Geometry: final body of the model. Coordinates: model frame, mm. Face numbers are marked on the shaded views. A direction names the side the tool comes from. Round coordinates to 2 decimals unless told otherwise and drop trailing zeros. Write each loop counter-clockwise with the first axis right and the second up, starting at its lowest first coordinate (ties: lowest second). Pieces come first, ordered by that corner, then holes.
from build123d import *

# Parameters (mm, degrees)
BOSS_EXTRUDE1_DEPTH = 25.5
CUT_EXTRUDE1_DEPTH  = 12.5
CUT_EXTRUDE2_DEPTH  = 15.75
BOSS_EXTRUDE2_REACH = 27.5
SKETCH2_W           = 6.25
SKETCH2_H           = 14
CUT_EXTRUDE3_DEPTH  = 9.5
FILLET1_R           = 8


with BuildPart() as part:
    # Sketch1 → Boss-Extrude1 (new body)
    with BuildSketch(Plane(origin=(0, 0, 0), x_dir=(1, 0, 0), z_dir=(0, 1, 0))):
        Polygon((0, 0), (44, 0), (44, -26), (34.5, -26), (34.5, -32), (0, -32), align=None)
    extrude(amount=BOSS_EXTRUDE1_DEPTH)

    # Sketch3 → Cut-Extrude1 (cut)
    with BuildSketch(Plane.ZY):
        Polygon((32, 25.5), (3.5, 25.5), (32, 9.5), align=None)
    extrude(amount=-CUT_EXTRUDE1_DEPTH, mode=Mode.SUBTRACT)

    # Sketch4 → Cut-Extrude2 (cut)
    with BuildSketch(Plane.ZY.offset(-12.5)):
        Polygon((32, 25.5), (3.5, 25.5), (32, 16), align=None)
    extrude(amount=-CUT_EXTRUDE2_DEPTH, mode=Mode.SUBTRACT)

    # Boss-Extrude2: up to this face of the body (flat: up to its plane)
    boss_extrude2_end = Plane(part.part.faces().sort_by_distance((20.375, 20.75, 17.75))[0])
    # Sketch2 → Boss-Extrude2 (add, up to the picked face)
    with BuildSketch(Plane(origin=(0, 25.5, 0), x_dir=(1, 0, 0), z_dir=(0, 1, 0)), mode=Mode.PRIVATE) as boss_extrude2_sk1:
        with Locations((15.625, -10.5)):
            Rectangle(SKETCH2_W, SKETCH2_H)
    boss_extrude2_tool1 = split(extrude(boss_extrude2_sk1.sketch, amount=-BOSS_EXTRUDE2_REACH, mode=Mode.PRIVATE), bisect_by=boss_extrude2_end, keep=Keep.BOTH, mode=Mode.PRIVATE)
    add(boss_extrude2_tool1.solids().sort_by_distance((15.625, 25.5, 10.5))[0])

    # Sketch5 → Cut-Extrude3 (cut)
    with BuildSketch(Plane(origin=(44, 0, 0), x_dir=(0, 0, -1), z_dir=(1, 0, 0))):
        with BuildLine():
            Line((-10.958518779, 18.837056558), (-3.5, 25.5))
            Line((-3.5, 25.5), (-26, 25.5))
            Line((-26, 25.5), (-26, 5.4))
            Line((-26, 5.4), (-20.653405287, 10.176291277))
            ThreePointArc((-20.653405287, 10.176291277), (-11.469613255, 9.652552152), (-10.958518779, 18.837056558))
        make_face()
    extrude(amount=-CUT_EXTRUDE3_DEPTH, mode=Mode.SUBTRACT)

    # Fillet1
    fillet1_edges = [part.edges().sort_by_distance(p)[0] for p in [
        (0, 4.75, 32),
    ]]
    fillet(fillet1_edges, radius=FILLET1_R)


solid = part.part
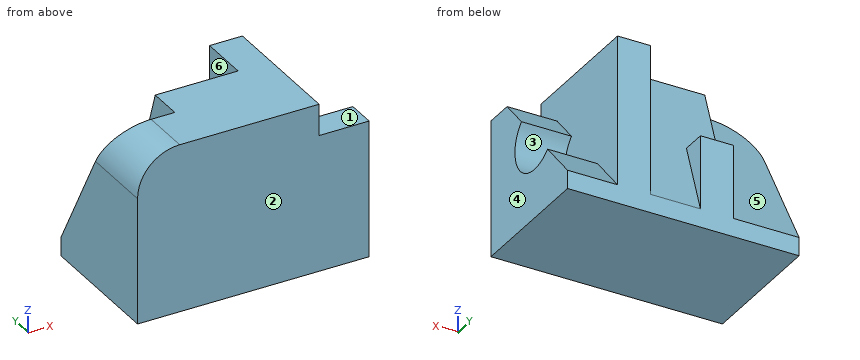
1) Reachability of the marked faces 4, 5 and 6 from +Z, -Z, +X, -X, +Y, -Y: full face, straight path, thin tool, end or side. Return the list, or none.
2) Section C-C on z = 15.8. Output: boundary loops of the cut face in (x, y), plus the area to 3 significant figures.
3) Line query: probe 1 along Z at (x, y) = (16, 21.75); probe 2 along X at (y, z) = (20, 18); probe 3 along X at (y, z) = (13, 11). Output: solid intervals per line, ascending.
4) Section B-B on y = 17.75. Output: boundary loops of the cut face in (x, z).
5) First-contact query: P1, Ø2.5, axis at y = 23, z = 9, coming from the +X side; P2, Ø3, axis at y = 21.5, z = 20, coming from the -X side; P3, Ø2.5, axis at x = 41.5, y = 1.5, coming from the +Z side. Flat tips, straight axial feed; report the tip coordinate or a pass-through.
6) Draft query along Z for the marked faces 1, 2 and 3. Return one class per face: pulls with the +Z half, pulls with the -Z half, needs draft (parallel to the pull), parting line crosses it, or undercut.
7) Section A-A on x = 16. Output: boundary loops of the cut face in (y, z).
Filled in:
1. face 4: +Z, -Z, +X, +Y, -Y
1. face 5: +Z, -X, +Y
1. face 6: +Z, +Y
2. outline: (0, 0) - (44, 0) - (44, 8) - (34.5, 8) - (34.5, 25.5) - (28.25, 25.5) - (28.25, 21.4) - (18.75, 21.4) - (18.75, 25.5) - (12.5, 25.5) - (12.5, 18.59) - (0, 18.59) - close
2. area: 830 mm2
3. probe 1: z = 0 to 17.5
3. probe 2: x = 12.5 to 34.5
3. probe 3: x = 0 to 34.5
4. outline: (0, 0) - (44, 0) - (44, 10.17) - (34.5, 10.17) - (34.5, 32) - (28.25, 32) - (28.25, 26.75) - (12.5, 26.75) - (12.5, 17.3) - (0, 17.3) - close
5. P1: stops at x = 34.5
5. P2: stops at x = 12.5
5. P3: stops at z = 26
6. face 1: pulls with the +Z half
6. face 2: needs draft
6. face 3: undercut
7. outline: (0, 0) - (25.5, 0) - (25.5, 17.5) - (20.83, 17.5) - (16, 32) - (0, 32) - close
